The model under review builds one solid part; all positions refer to its coordinate system, in mm. Face numbers are marked on the shaded views. A direction names the side the tool comes from. Coordinates: 2 decimals unless noted, no trailing zeros. Loops run counter-clockwise (first coordinate to the right, second up) from the corner with the lowest first, then second, coordinate; pieces in that order, holes last. Notation, with made-up numbers: (33.25, 28) - (46.25, 28) arc R32 cw to (46.25, 55) - close; hole circle Ø9 at (82, -35.75). An arc over 180 degrees is marked (long way). One line per item, written item: value. Start each with the question number.
1. For the marked faces 4 and 5, list the 3-axis set-ups (+Z, -Z, +X, -X, +Y, -Y) from which the entire face can be reached by the end or side of a thin tool; tool diameter is ignored.
2. We need section D-D, the plane z = -3. Give the boundary of the cut face in (x, y).
3. We need section A-A, the plane x = 0. Give the boundary of the cut face in (y, z).
4. We need section C-C, the plane x = 3. Give the boundary of the cut face in (y, z), then the cut area to 3 significant figures.
5. Mouldability with a two-part tool opening along Z and no side actions: class the marked faces 1, 2 and 3 as +Z half, -Z half, draft (parallel to the pull), parting line (faces both ways), or undercut.
6. We need section B-B, the plane y = 9.5. Give the boundary of the cut face in (x, z), then the cut area to 3 significant figures.
7. To check wall thickness, follow line 1 (X direction, y = 6, z = 0); line 2 (Z direction, x = 0.5, y = 4); line 3 (Y direction, x = -2, z = 5.5). State the ranges of each line that lie inside material, in increasing order.
8. Insertion check: P1, Ø3.5, axis at y = 5, z = -7.81, coming from the -X side; P2, Ø4.5, axis at x = 2.5, y = 12.5, coming from the +Z side. Each pin has a flat end and moves straight along its axis. Give the tip position at first contact, or say it passes through.
from build123d import *

# Parameters (mm, degrees)
SKETCH1_W                = 12
SKETCH1_H                = 23.373361116
SKETCH1_R                = 2
BOSS_EXTRUDE1_DEPTH      = 10
BOSS_EXTRUDE2_DEPTH      = 4
BOSS_EXTRUDE2_DEPTH_BACK = 10
SKETCH2_W                = 12
SKETCH2_H                = 3
SKETCH3_R                = 2
CUT_EXTRUDE1_DEPTH       = 14


with BuildPart() as part:
    # Sketch1 → Boss-Extrude1 (new body)
    with BuildSketch(Plane(origin=(0, 0, 0), x_dir=(1, 0, 0), z_dir=(0, 1, 0))):
        with Locations((0, 3.313319442)):
            Rectangle(SKETCH1_W, SKETCH1_H)
        with Locations(Location((0, 0, 0), (0, 0, 270))):
            Circle(SKETCH1_R, mode=Mode.SUBTRACT)
    extrude(amount=BOSS_EXTRUDE1_DEPTH)

    # Sketch2 → Boss-Extrude2 (add, two sides: drawn at the far end of the back side and taken through both)
    with BuildSketch(Plane(origin=(0, 10, 0), x_dir=(1, 0, 0), z_dir=(0, 1, 0)).offset(-BOSS_EXTRUDE2_DEPTH_BACK)):
        with Locations((0, 16.5)):
            Rectangle(SKETCH2_W, SKETCH2_H)
    extrude(amount=BOSS_EXTRUDE2_DEPTH + BOSS_EXTRUDE2_DEPTH_BACK)

    # Sketch3 → Cut-Extrude1 (cut)
    with BuildSketch(Plane.ZY.offset(6)):
        with Locations((-7.813319442, 5)):
            Circle(SKETCH3_R)
        with Locations((-1.813319442, 5)):
            Circle(SKETCH3_R)
    extrude(amount=-CUT_EXTRUDE1_DEPTH, mode=Mode.SUBTRACT)


solid = part.part
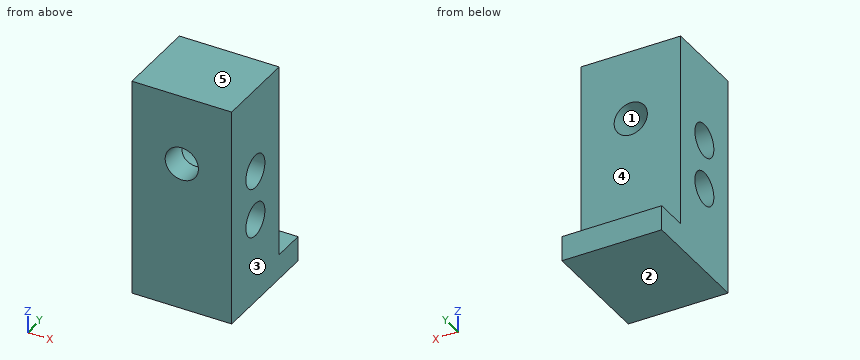
Findings below:
1. face 4: +Z, +X, -X, +Y
1. face 5: +Z, +X, -X, +Y, -Y
2. outline: (-6, 0) - (6, 0) - (6, 3.39) - (-6, 3.39) - close; (-6, 6.61) - (6, 6.61) - (6, 10) - (-6, 10) - close
3. outline: (0, -18) - (14, -18) - (14, -15) - (10, -15) - (10, -2) - (6.99, -2) arc R2 cw to (3.01, -2) - (0, -2) - close; (0, 2) - (10, 2) - (10, 8.37) - (0, 8.37) - close; hole circle Ø4 at (5, -7.81)
4. outline: (0, -18) - (14, -18) - (14, -15) - (10, -15) - (10, 8.37) - (0, 8.37) - close; hole circle Ø4 at (5, -7.81); hole circle Ø4 at (5, -1.81)
4. area: 251 mm2
5. face 1: undercut
5. face 2: -Z half
5. face 3: draft
6. outline: (-6, -18) - (6, -18) - (6, 8.37) - (-6, 8.37) - close; hole circle Ø4 at (0, 0)
6. area: 304 mm2
7. line 1: -6 to -2, 2 to 6
7. line 2: -18 to -9.55, -6.08 to -3.55, 1.94 to 8.37
7. line 3: 0 to 10
8. P1: through
8. P2: z = -15
